from build123d import *

# Parameters (mm, degrees)
SKETCH_1_W          = 50
SKETCH_1_H          = 100
EXTRUDE_1_DEPTH     = 17.2
FILLET_1_R          = 15
CUT_EXTRUDE_3_DEPTH = 26
SKETCH_6_R          = 3
CUT_EXTRUDE_4_DEPTH = 114.11869872
CUT_EXTRUDE_5_DEPTH = 114.11869872
FILLET_2_R          = 6
FILLET_3_R          = 6
SKETCH_9_R          = 3
CUT_EXTRUDE_6_DEPTH = 114.11869872
SKETCH_10_R         = 6
CUT_EXTRUDE_7_DEPTH = 9


with BuildPart() as part:
    # Эскиз1 → Бобышка-Вытянуть1 (new body)
    with BuildSketch(Plane.XY):
        with Locations((25, 50)):
            Rectangle(SKETCH_1_W, SKETCH_1_H)
    extrude(amount=EXTRUDE_1_DEPTH)

    # Скругление1
    fillet_1_edges = [part.edges().sort_by_distance(p)[0] for p in [
        (25, 100, 17.2),
        (25, 0, 17.2),
    ]]
    fillet(fillet_1_edges, radius=FILLET_1_R)

    # Эскиз5 → Вырез-Вытянуть3 (cut)
    with BuildSketch(Plane(origin=(0, 37, 0), x_dir=(1, 0, 0), z_dir=(0, 1, 0))):
        Polygon((0, -17.2), (0, -12), (15, -17.2), align=None)
    extrude(amount=CUT_EXTRUDE_3_DEPTH, mode=Mode.SUBTRACT)

    # Эскиз6 → Вырез-Вытянуть4 (cut, through all)
    with BuildSketch(Plane.XY.offset(17.2)):
        with Locations((25, 50)):
            Circle(SKETCH_6_R)
    extrude(amount=-CUT_EXTRUDE_4_DEPTH, mode=Mode.SUBTRACT)

    # Эскиз7 → Вырез-Вытянуть5 (cut, through all)
    with BuildSketch(Plane(origin=(0, 0, 0), x_dir=(-1, 0, 0), z_dir=(0, 0, -1))):
        Polygon((0, 57), (0, 43), (-13.646386899, 47), (-25, 47), (-25, 53), (-13.646386899, 53), align=None)
    extrude(amount=-CUT_EXTRUDE_5_DEPTH, mode=Mode.SUBTRACT)

    # Скругление2
    fillet_2_edges = [part.edges().sort_by_distance(p)[0] for p in [
        (0, 57, 6),
        (0, 43, 6),
    ]]
    fillet(fillet_2_edges, radius=FILLET_2_R)

    # Скругление3
    fillet_3_edges = [part.edges().sort_by_distance(p)[0] for p in [
        (13.646386899, 53, 8.365373729),
        (13.646386899, 47, 8.365373729),
    ]]
    fillet(fillet_3_edges, radius=FILLET_3_R)

    # Эскиз9 → Вырез-Вытянуть6 (cut, through all)
    with BuildSketch(Plane(origin=(0, 0, 0), x_dir=(-1, 0, 0), z_dir=(0, 0, -1))):
        with Locations((-40, 29.35)):
            Circle(SKETCH_9_R)
        with Locations((-10, 29.35)):
            Circle(SKETCH_9_R)
        with Locations((-10, 70.65)):
            Circle(SKETCH_9_R)
        with Locations((-40, 70.65)):
            Circle(SKETCH_9_R)
    extrude(amount=-CUT_EXTRUDE_6_DEPTH, mode=Mode.SUBTRACT)

    # Эскиз10 → Вырез-Вытянуть7 (cut)
    with BuildSketch(Plane(origin=(0, 0, 0), x_dir=(-1, 0, 0), z_dir=(0, 0, -1))):
        with Locations((-40, 29.35)):
            Circle(SKETCH_10_R)
        with Locations((-10, 29.35)):
            Circle(SKETCH_10_R)
        with Locations((-10, 70.65)):
            Circle(SKETCH_10_R)
        with Locations((-40, 70.65)):
            Circle(SKETCH_10_R)
    extrude(amount=-CUT_EXTRUDE_7_DEPTH, mode=Mode.SUBTRACT)


solid = part.part
Geometry check sheet. Reference: the model listing, model coordinates, mm. A direction names the side the tool comes from. Give positions to 0.01 mm unless a question says otherwise; leave off trailing zeros. Write each loop counter-clockwise with the first axis right and the second up, starting at its lowest first coordinate (ties: lowest second). Pieces come first, ordered by that corner, then holes. Notation, with made-up numbers: M -23.5,33 L -8.5,33 A28 ccw -8.5,65 Z; hole C -17.75,77 d9. An arc over 180 degrees is marked long. Answer as CSV lines item,"result". Start each with the question number.
Q1. Section check C-C, the plane x = 40. Record the cut outline in (y, z).
Q2. Tool access check on faces 4 (the face through (10.78, 76.6, 4.44)), 5 (the face through (7.395, 40.819, 14.564)), 6 (the face through (25.35, 95.72, 12.69)), 7 (the face through (20, 47, 8)). Record the directions out of +Z, -Z, +X, -X, +Y, -Y that give a thin tool (end or side, any length) a straight path to the whole face; none if there is none.
Q3. Section check A-A, the plane x = 20. Record the cut outline in (y, z).
Q4. Go/stop test with flat-tipped pins: pin 1 (1.6 mm diameter, centred on x = 5, z = 15, fed in from -Y); pin 2 (5 mm diameter, centred on x = 41, z = 6, fed in from -Y); pin 3 (3 mm diameter, centred on x = 24, z = 10, fed in from -Y). Record where each tip stops, or that it passes through.
Q5. Release check for a two-part mould opening along X. For faces 1 (the face through (1.165, 42.06, 6.842)), 2 (the face through (13, 28, 9)), 3 (the face through (4, 37, 16)) record: pulls with the +X half, pulls with the -X half, needs draft (parallel to the pull), parting line crosses it, or undercut.
Q6. Section check D-D, the plane z = 6. Record the cut outline in (x, y).
Q7. Section check B-B, the plane y = 29.35. Record the cut outline in (x, z), then the cut area to 3 significant figures.
Q8. Material ranges on L1, parallel to Y at x = 40, z = 14.75; L2, parallel to Y at x = 40, z = 3.5; L3, parallel to Y at x = 2, z = 3.5, recorded low to high.
Geometry says:
1,outline,"M 0,0 L 23.35,0 L 23.35,9 L 26.35,9 L 26.35,17.2 L 15,17.2 A15 ccw 0,2.2 Z; M 32.35,9 L 35.35,9 L 35.35,0 L 64.65,0 L 64.65,9 L 67.65,9 L 67.65,17.2 L 32.35,17.2 Z; M 73.65,9 L 76.65,9 L 76.65,0 L 100,0 L 100,2.2 A15 ccw 85,17.2 L 73.65,17.2 Z"
2,face 4,"-Z"
2,face 5,"+Z, -X"
2,face 6,"+Z, +X, -X, +Y"
2,face 7,"+Z, -Z, -X"
3,outline,"M 0,0 L 47,0 L 47,17.2 L 15,17.2 A15 ccw 0,2.2 Z; M 53,0 L 100,0 L 100,2.2 A15 ccw 85,17.2 L 53,17.2 Z"
4,pin 1,"y = 6"
4,pin 2,"y = 0.06"
4,pin 3,"y = 1.39"
5,face 1,"pulls with the -X half"
5,face 2,"undercut"
5,face 3,"needs draft"
6,outline,"M 0,0.49 L 50,0.49 L 50,99.51 L 0,99.51 L 0,61.49 A6 ccw 4.31,55.74 L 12.82,53.24 A6 ccw 14.51,53 L 25,53 A3 cw 25,47 L 14.51,47 A6 ccw 12.82,46.76 L 4.31,44.26 A6 ccw 0,38.51 Z; hole C 10,29.35 d12; hole C 10,70.65 d12; hole C 40,29.35 d12; hole C 40,70.65 d12"
7,outline,"M 0,0 L 4,0 L 4,9 L 7,9 L 7,17.2 L 0,17.2 Z; M 13,9 L 16,9 L 16,0 L 34,0 L 34,9 L 37,9 L 37,17.2 L 13,17.2 Z; M 43,9 L 46,9 L 46,0 L 50,0 L 50,17.2 L 43,17.2 Z"
7,area,"546 mm^2"
8,L1,"6.78 to 26.35, 32.35 to 67.65, 73.65 to 93.22"
8,L2,"0.06 to 23.35, 35.35 to 64.65, 76.65 to 99.94"
8,L3,"0.06 to 42.98, 57.02 to 99.94"
